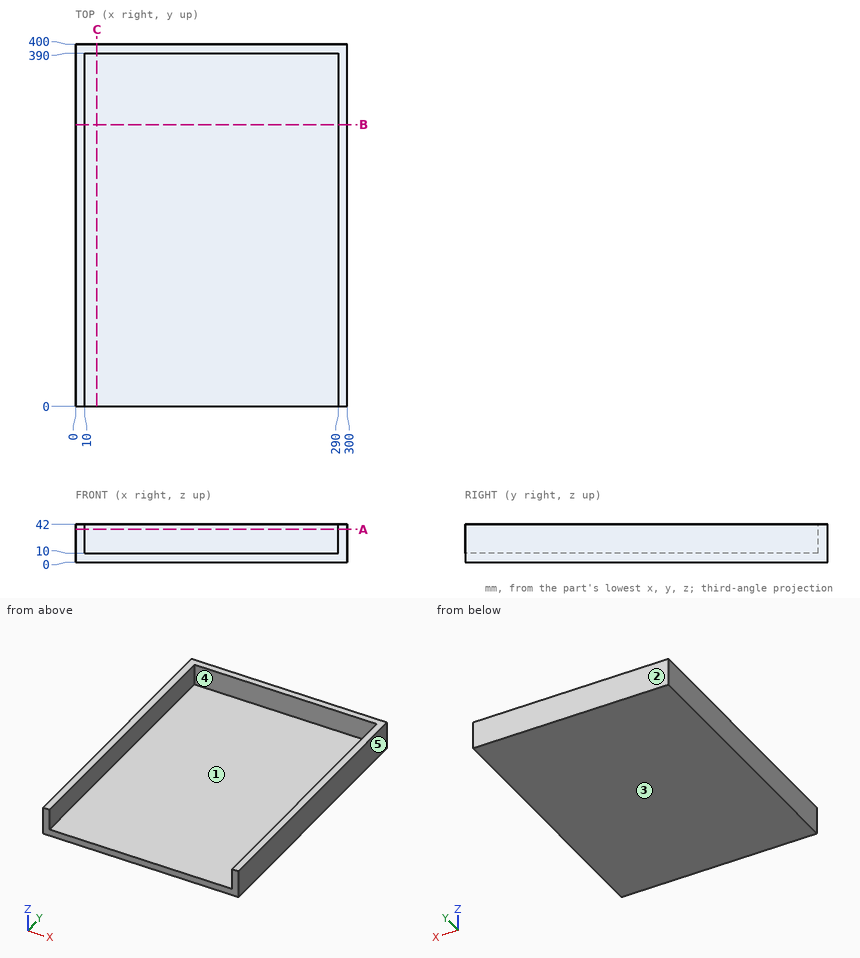
Here's the drawing with two shaded views (mm, measured from the low corner). I have some questions. A direction names the side the tool comes from. Give positions to 0.01 mm unless a question says otherwise; leave off trailing zeros. Write each loop counter-clockwise with the first axis right and the second up, starting at its lowest first coordinate (ties: lowest second). Pieces come first, ordered by that corner, then holes. Notation, with made-up numbers: (-8.75, 28.25) -> (14.25, 28.25) arc R22 cw to (14.25, 35.25) -> close; hole circle Ø7 at (21.25, -33.5). An arc over 180 degrees is marked (long way). Answer as a JSON object with one key per item and string values. Group by question number.
Item 1: Suppose I cut it at A-A (z = 36.5). Please give me the cut outline in (x, y).
Item 2: We'd pull the mould along X, two halves only. Please class the marked faces 3, 4 and 5: +X half, -X half, draft (parallel to the pull), parting line (faces both ways), or undercut.
Item 3: Suppose I cut it at C-C (x = 23.5). Please give me the cut outline in (y, z), plus the area to 3 significant figures.
Item 4: For the marked faces 1 and 2, which set-ups out of +Z, -Z, +X, -X, +Y, -Y let a thin tool reach every point of the face, with its end or its side?
Item 5: I'm going to push flat-ended pins straight in: P1, Ø1.5, axis at x = 215.5, y = 52.5, coming from the +Z side; P2, Ø12, axis at x = 267.5, z = 27, coming from the -Y side. Where does each tip first touch, or does it pass through?
Item 6: Suppose I cut it at B-B (y = 311). Please give me the cut outline in (x, z).
Item 7: Please list where these lines run through material, in increasing order: line 1 (X direction, y = 208, z = 13); line 2 (Z direction, x = 55, y = 258); line 3 (Y direction, x = 14, z = 17). Write a range as [from, to].
Findings:
{
 "1": {"outline": "(0, 0) -> (10, 0) -> (10, 390) -> (290, 390) -> (290, 0) -> (300, 0) -> (300, 400) -> (0, 400) -> close"},
 "2": {"face 3": "draft", "face 4": "undercut", "face 5": "+X half"},
 "3": {"outline": "(0, 0) -> (400, 0) -> (400, 42) -> (390, 42) -> (390, 10) -> (0, 10) -> close", "area": "4,320 mm²"},
 "4": {"face 1": "+Z, -Y", "face 2": "+Z, -Z, +X, -X, +Y"},
 "5": {"P1": "stops at z = 10", "P2": "stops at y = 390"},
 "6": {"outline": "(0, 0) -> (300, 0) -> (300, 42) -> (290, 42) -> (290, 10) -> (10, 10) -> (10, 42) -> (0, 42) -> close"},
 "7": {"line 1": "x = [0, 10], [290, 300]", "line 2": "z = [0, 10]", "line 3": "y = [390, 400]"}
}
